Can you work these out from the model? Positions are in its coordinate system, mm. Round coordinates to 2 decimals unless told otherwise and drop trailing zeros. Loops run counter-clockwise (first coordinate to the right, second up) from the corner with the lowest first, then second, coordinate; pieces in that order, holes last. Notation, with made-up numbers: (76.25, 39.25) -> (84.25, 39.25) arc R34 cw to (84.25, 78.25) -> close; hole circle Ø8 at (5.5, 50.25). An arc over 180 degrees is marked (long way). Write each question's results on one line, items separated by ' | '.
from build123d import *

# Parameters (mm, degrees)
SKETCH_1_R          = 115
EXTRUDE_1_DEPTH     = 10
SKETCH_2_R          = 104
EXTRUDE_2_DEPTH     = 15
CHAMFER_1_SIZE      = 1
CHAMFER_2_SIZE      = 2
SKETCH_3_R          = 8.5
CUT_EXTRUDE_1_DEPTH = 25


with BuildPart() as part:
    # Эскиз1 → Бобышка-Вытянуть1 (new body)
    with BuildSketch(Plane(origin=(0, 0, 0), x_dir=(1, 0, 0), z_dir=(0, 1, 0))):
        Circle(SKETCH_1_R)
    extrude(amount=EXTRUDE_1_DEPTH)

    # Эскиз2 → Бобышка-Вытянуть2 (add)
    with BuildSketch(Plane(origin=(0, 10, 0), x_dir=(1, 0, 0), z_dir=(0, 1, 0))):
        Circle(SKETCH_2_R)
    extrude(amount=EXTRUDE_2_DEPTH)

    # Фаска1
    chamfer_1_edges = [part.edges().sort_by_distance(p)[0] for p in [
        (-115, 0, 0),
        (-115, 10, 0),
    ]]
    chamfer(chamfer_1_edges, length=CHAMFER_1_SIZE)

    # Фаска2
    chamfer_2_edges = [part.edges().sort_by_distance(p)[0] for p in [
        (-104, 25, 0),
    ]]
    chamfer(chamfer_2_edges, length=CHAMFER_2_SIZE)

    # Эскиз3 → Вырез-Вытянуть1 (cut)
    with BuildSketch(Plane(origin=(0, 25, 0), x_dir=(1, 0, 0), z_dir=(0, 1, 0))):
        Circle(SKETCH_3_R)
    extrude(amount=-CUT_EXTRUDE_1_DEPTH, mode=Mode.SUBTRACT)


solid = part.part
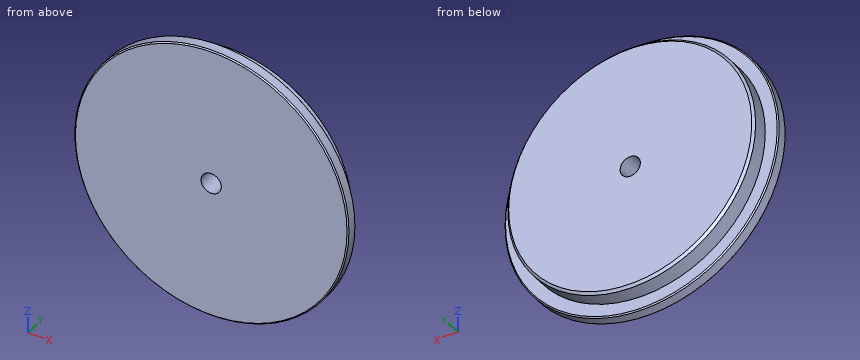
1. Please list where these lines run through material, in increasing order: line 1 (X direction, y = 11.75, z = 0); line 2 (Z direction, x = 0, y = 6). Write a range as from..to.
Final values:
line 1: -104..-8.5, 8.5..104 | line 2: -115..-8.5, 8.5..115
2. Will these pins go through, and if not, where does the flat tip stop? pin 1 (8 mm diameter, centred on y = 16.5, z = -45.5, fed in from -X); pin 2 (5 mm diameter, centred on x = -24, y = 10.5, fed in from -Z); pin 3 (1 mm diameter, centred on y = 15, z = 55.5, fed in from -X).
Final values:
pin 1: x = -95.36 | pin 2: z = -112.88 | pin 3: x = -88.27
3. If we section it at B-B (x = 0): List the corners of the cut face in (y, z) for me.
Final values:
outline: (0, -114) -> (1, -115) -> (9, -115) -> (10, -114) -> (10, -104) -> (23, -104) -> (25, -102) -> (25, -8.5) -> (0, -8.5) -> close; (0, 8.5) -> (25, 8.5) -> (25, 102) -> (23, 104) -> (10, 104) -> (10, 114) -> (9, 115) -> (1, 115) -> (0, 114) -> close
4. If we section it at C-C (y = 16): List the corners of the cut face in (x, z) for me.
Final values:
outline: circle Ø208 at (0, 0); hole circle Ø17 at (0, 0)
5. If we section it at A-A (z = 0): List the corners of the cut face in (x, y) for me, then the cut area to 3 significant figures.
Final values:
outline: (-115, 1) -> (-114, 0) -> (-8.5, 0) -> (-8.5, 25) -> (-102, 25) -> (-104, 23) -> (-104, 10) -> (-114, 10) -> (-115, 9) -> close; (8.5, 0) -> (114, 0) -> (115, 1) -> (115, 9) -> (114, 10) -> (104, 10) -> (104, 23) -> (102, 25) -> (8.5, 25) -> close | area: 4,990 mm2
